```python
from build123d import *

# Parameters (mm, degrees)
F1_DEPTH = 50
F2_SIZE  = 5
F3_W     = 20
F3_H     = 20
F4_DEPTH = 10
F5_R     = 5
F6_DEPTH = 100


with BuildPart() as f1:
    # F0 (on Front) → F1 (new body, symmetric)
    with BuildSketch(Plane.XZ):
        with BuildLine():
            Line((40, -20), (40, 20))
            Line((40, 20), (-40, 20))
            Line((-40, 20), (-40, -20))
            Line((-40, -20), (-35, -20))
            Line((-35, -20), (-35, 10))
            ThreePointArc((-35, 10), (-33.535534, 13.535534), (-30, 15))
            Line((-30, 15), (30, 15))
            ThreePointArc((30, 15), (33.535534, 13.535534), (35, 10))
            Line((35, 10), (35, -20))
            Line((35, -20), (40, -20))
        make_face()
    extrude(amount=F1_DEPTH, both=True)

    # F2
    f2_edges = [f1.edges().sort_by_distance(p)[0] for p in [
        (40, 0, 20),
        (-40, 0, 20),
    ]]
    chamfer(f2_edges, length=F2_SIZE)

    # F3 (on face) → F4 (cut)
    with BuildSketch(Plane.XY.offset(20)):
        with Locations((0, 14.830591)):
            Rectangle(F3_W, F3_H)
    extrude(amount=-F4_DEPTH, mode=Mode.SUBTRACT)

    # F5 (on face) → F6 (cut)
    with BuildSketch(Plane.YZ.offset(40)):
        with Locations((-30, 0)):
            Circle(F5_R)
    extrude(amount=-F6_DEPTH, mode=Mode.SUBTRACT)


solid = f1.part
```
Input: part model. Units: mm. Frame: model coordinates. A direction names the side the tool comes from. Round coordinates to 2 decimals unless told otherwise and drop trailing zeros. Loops run counter-clockwise (first coordinate to the right, second up) from the corner with the lowest first, then second, coordinate; pieces in that order, holes last. Notation, with made-up numbers: (87, -40) - (92, -40) arc R20 cw to (92, -34) - close; hole circle Ø7 at (2.25, 41.25). An arc over 180 degrees is marked (long way). One line per item, written item: value. Start each with the question number.
(1) Section D-D, the plane z = 0. Return loops of the section in (x, y).
(2) Section B-B, the plane z = 8. Return loops of the section in (x, y), plus the area to 3 significant figures.
(3) Access query for faces 5 (the flat face through (37, -1, -20)), 6 (the cylindrical face through (-34, -1, 13)), 7 (the flat face through (10, 15, 18)). Directions: +Z, -Z, +X, -X, +Y, -Y. A direction counts if a zero-diameter tool reaches every point of the face in a straight line with its end or side. Return the directions, or none.
(4) Ray query, line 1 (X direction, y = -19, z = 5); line 2 (Z direction, x = -12.5, y = -29); line 3 (X direction, y = -31, z = 12.5). Return the intervals inside material, ascending. Write a range as [from, to].
(5) Section A-A, the plane y = -30. Return loops of the section in (x, z).
(6) Section C-C, the plane x = 7.5. Return loops of the section in (y, z).
(7) Contact query for flat-ended pins moving along their axis: P1, Ø2.5, axis at y = 18.5, z = 17.5, coming from the -X side; P2, Ø11.5, axis at y = -30, z = 0, coming from the +X side; P3, Ø18, axis at x = 3.5, y = -2.5, coming from the -Z side; P4, Ø1.5, axis at y = 12, z = 18.5, coming from the +X side. Output: stop coordinate, or through.
(8) Draft query along Y for faces 1 (the flat face through (-3, -50, 16)), 2 (the flat face through (-37, 1, 18)), 3 (the flat face through (-3, 50, 16)), 4 (the cylindrical face through (38, -35, 0)). Return one class per face: +Y half, -Y half, draft (parallel to the pull), parting line (faces both ways), or undercut.
Results below:
1. outline: (-40, -50) - (-35, -50) - (-35, -35) - (-40, -35) - close; (-40, -25) - (-35, -25) - (-35, 50) - (-40, 50) - close; (35, -50) - (40, -50) - (40, -35) - (35, -35) - close; (35, -25) - (40, -25) - (40, 50) - (35, 50) - close
2. outline: (-40, -50) - (-35, -50) - (-35, 50) - (-40, 50) - close; (35, -50) - (40, -50) - (40, 50) - (35, 50) - close
2. area: 1,000 mm^2
3. face 5: -Z, +X, -X, +Y, -Y
3. face 6: -Z, +Y, -Y
3. face 7: +Z, -Z
4. line 1: [-40, -35], [35, 40]
4. line 2: [15, 20]
4. line 3: [-40, -34.33], [34.33, 40]
5. outline: (-40, -20) - (-35, -20) - (-35, -5) - (-40, -5) - close; (-40, 5) - (-35, 5) - (-35, 10) arc R5 cw to (-30, 15) - (30, 15) arc R5 cw to (35, 10) - (35, 5) - (40, 5) - (40, 15) - (35, 20) - (-35, 20) - (-40, 15) - close; (35, -20) - (40, -20) - (40, -5) - (35, -5) - close
6. outline: (-50, 15) - (4.83, 15) - (4.83, 20) - (-50, 20) - close; (24.83, 15) - (50, 15) - (50, 20) - (24.83, 20) - close
7. P1: x = -38.75
7. P2: x = 40
7. P3: z = 15
7. P4: x = 37.25
8. face 1: -Y half
8. face 2: draft
8. face 3: +Y half
8. face 4: undercut
